```python
from build123d import *

# Parameters (mm, degrees)
F1_DEPTH = 6.1
F2_DEPTH = 0.65
F3_W     = 6.35
F3_H     = 3.35
F4_DEPTH = 1
F5_W     = 6.35
F5_H     = 3.35
F6_DEPTH = 1
F7_ANGLE = 180
F8_DEPTH = 1


with BuildPart() as f1:
    # F0 (on Front) → F1 (new body, symmetric)
    with BuildSketch(Plane.XZ):
        Polygon((-3.2191018649, 0), (-2.2191018649, 0), (-2.2191018649, 2.65), (-1.6191018649, 2.65), (-1.6191018649, 3), (2.1308981351, 3), (2.1308981351, 0), (3.1308981351, 0), (3.1308981351, 4), (-3.2191018649, 4), align=None)
    extrude(amount=F1_DEPTH, both=True)

    # F2 (cut): a face of the model
    f2_faces = [f1.faces().sort_by_distance(p)[0] for p in [
        (-2.7191018649, 0, 0),
    ]]
    extrude(f2_faces, amount=-F2_DEPTH, mode=Mode.SUBTRACT)

    # F3 (on face) → F4 (join)
    with BuildSketch(Plane.XZ.offset(6.1)):
        with Locations((-0.0441018649, 2.325)):
            Rectangle(F3_W, F3_H)
    extrude(amount=F4_DEPTH)

    # F5 (on face) → F6 (join)
    with BuildSketch(Plane(origin=(0, 6.1, 0), x_dir=(-1, 0, 0), z_dir=(0, 1, 0))):
        with Locations((0.0441018649, 2.325)):
            Rectangle(F5_W, F5_H)
    extrude(amount=F6_DEPTH)


with BuildPart() as f1_1:
    # F7: moved
    add(f1.part.rotate(Axis((-0.0441018649, -7.1, 0.65), (1, 0, 0)), F7_ANGLE))

    # F8 (cut, through all): a face of the model
    f8_faces = [f1_1.faces().sort_by_distance(p)[0] for p in [
        (-2.2191018649, -14.2, -0.35),
    ]]
    extrude(f8_faces, amount=-F8_DEPTH, mode=Mode.SUBTRACT)


solid = f1_1.part
```
CAD build for the part. Positions are in the model's coordinates, mm. A direction names the side the tool comes from. Coordinates: 2 decimals unless noted, no trailing zeros. Order: outer loops, then holes, each group sorted by start corner. A loop starts at its lowest first (then second) coordinate and runs counter-clockwise, first axis right, second up.
(1) Which spindle directions (+Z, -Z, +X, -X, +Y, -Y) get a long thin tool onto all of the face, cutting with end or side? Do faces 5 (the face through (-3.219, -14, -2)), 6 (the face through (0, -14, -1.7)). Say none if no direction does.
Solution:
face 5: +Z, -Z, -X, +Y, -Y
face 6: +Z
(2) Saw through at A-A, the plane y = -11.75. Write the cut outline in (x, z), and give its area (3 significant figures).
Solution:
outline: (-3.22, -2.7) - (3.13, -2.7) - (3.13, 1.3) - (2.13, 1.3) - (2.13, -1.7) - (-1.62, -1.7) - (-1.62, -1.35) - (-3.22, -1.35) - close
area: 9.91 mm2
(3) Drill centre lines: L1, parallel to Y at x = -0.75, z = -0.6; L2, parallel to X at y = -16.75, z = -1.45; L3, parallel to Z at x = -0.5, y = -18.75. Where is each one in solid material? Low to high.
Solution:
L1: y = -21.3 to -20.3, -8.1 to -7.1
L2: x = -3.22 to -1.62, 2.13 to 3.13
L3: z = -2.7 to -1.7
(4) Mould opens along Y. For faces 1 (the face through (2.6, -14.1, 1.3)), 2 (the face through (-1, -8.1, -1)), 3 (the face through (0, -7.1, -1)), 4 (the face through (-2, -14, -1.35)) say: released by +Y, released by -Y, zero draft, split by the parting line, or undercut.
Solution:
face 1: zero draft
face 2: undercut
face 3: released by +Y
face 4: undercut
(5) Saw through at C-C, the plane y = -7.75. Write the cut outline in (x, z).
Solution:
outline: (-3.22, -2.7) - (3.13, -2.7) - (3.13, 0.65) - (-3.22, 0.65) - close
(6) Saw through at B-B, the plane x = 1. Write the cut outline in (y, z), and give its area (3 significant figures).
Solution:
outline: (-21.3, -2.7) - (-7.1, -2.7) - (-7.1, 0.65) - (-8.1, 0.65) - (-8.1, -1.7) - (-20.3, -1.7) - (-20.3, 0.65) - (-21.3, 0.65) - close
area: 18.9 mm2
(7) Pin check, flat tips, straight feed: pin 1 Ø0.5 at (x, y) = (-0.5, -21) entering from +Z; pin 2 Ø0.8 at (x, y) = (-3, -13) entering from +Z; pin 3 Ø0.8 at (x, y) = (1.5, -7.5) entering from +Z. Stop position of each tip, or through.
Solution:
pin 1: stops at z = 0.65
pin 2: stops at z = -1.35
pin 3: stops at z = 0.65
